Part model, mm, in its own coordinate system. A direction names the side the tool comes from. Round coordinates to 2 decimals unless told otherwise and drop trailing zeros. Loops run counter-clockwise (first coordinate to the right, second up) from the corner with the lowest first, then second, coordinate; pieces in that order, holes last.
(1) Cut at C-C on z = 16.5. List the corners of the cut face in (x, y).
(2) Cut at A-A on x = 21.5. List the corners of the cut face in (y, z).
(3) Tool access for faces 5 (the face through (37, 246, 41.5)), 6 (the face through (3, 500, -3)): list every direction of +Z, -Z, +X, -X, +Y, -Y with a clear straight run to the whole face (end or side of a thin tool).
(4) Probe probe 1 along Z at (x, y) = (29, 441); probe 2 along X at (y, z) = (414, -23.5); probe 3 along X at (y, z) = (424.5, 33.5). List the from-to ranges inside material, lowest first.
(5) Cut at B-B on y = 297. List the corners of the cut face in (x, z), then the cut area to 3 significant figures.
(6) Mould opens along Z. For faces 1 (the face through (7.706, 246.5, -38.934)), 2 (the face through (5, 246, 0)), 3 (the face through (30, 246, 50)), 4 (the face through (60, 246, 46)) say: +Z half, -Z half, draft (parallel to the pull), parting line (faces both ways), or undercut.
from build123d import *

# Parameters (mm, degrees)
F2_DEPTH = 500


with BuildPart() as f2:
    # F0 (on Front) → F2 (new body)
    with BuildSketch(Plane.XZ):
        with BuildLine():
            Line((0, 50), (0, 0))
            Line((0, 0), (0, -50))
            Line((0, -50), (60, -50))
            Line((60, -50), (60, -41.5))
            Line((60, -41.5), (14, -41.5))
            ThreePointArc((14, -41.5), (7.6360389693, -38.8639610307), (5, -32.5))
            Line((5, -32.5), (5, 0))
            Line((5, 0), (5, 32.5))
            ThreePointArc((5, 32.5), (7.6360389693, 38.8639610307), (14, 41.5))
            Line((14, 41.5), (60, 41.5))
            Line((60, 41.5), (60, 50))
            Line((60, 50), (0, 50))
        make_face()
    extrude(amount=-F2_DEPTH)


solid = f2.part
Final values:
1. outline: (0, 0) - (5, 0) - (5, 500) - (0, 500) - close
2. outline: (0, -50) - (500, -50) - (500, -41.5) - (0, -41.5) - close; (0, 41.5) - (500, 41.5) - (500, 50) - (0, 50) - close
3. face 5: +X, +Y, -Y
3. face 6: +Z, -Z, +X, -X, +Y
4. probe 1: z = -50 to -41.5, 41.5 to 50
4. probe 2: x = 0 to 5
4. probe 3: x = 0 to 5.06
5. outline: (0, -50) - (60, -50) - (60, -41.5) - (14, -41.5) arc R9 cw to (5, -32.5) - (5, 32.5) arc R9 cw to (14, 41.5) - (60, 41.5) - (60, 50) - (0, 50) - close
5. area: 1,470 mm2
6. face 1: undercut
6. face 2: undercut
6. face 3: +Z half
6. face 4: draft
